Here's how the part is built. I have some questions about the finished solid (model axes, mm). A direction names the side the tool comes from. Coordinates: 2 decimals unless noted, no trailing zeros. Write each loop counter-clockwise with the first axis right and the second up, starting at its lowest first coordinate (ties: lowest second). Pieces come first, ordered by that corner, then holes. Notation, with made-up numbers: (76, -20.75) -> (120, -20.75) arc R9 ccw to (120, -9.75) -> close; hole circle Ø3 at (-26.75, -20). An arc over 180 degrees is marked (long way). Use CSV: the item, a comma, the result in double quotes. Start each with the question number.
```python
from build123d import *

# Parameters (mm, degrees)
SKETCH1_W               = 88.9
SKETCH1_H               = 40
BOSS_EXTRUDE1_DEPTH     = 20
SKETCH2_R               = 5
CUT_EXTRUDE1_DEPTH      = 89.9
SKETCH3_R               = 5.6
CUT_EXTRUDE2_DEPTH      = 10
SKETCH4_R               = 4
CUT_EXTRUDE3_DEPTH      = 10
F_1_4_20_TAPPED_HOLE1_D = 5.1054
CHAMFER1_SIZE           = 1


with BuildPart() as part:
    # Sketch1 → Boss-Extrude1 (new body)
    with BuildSketch(Plane(origin=(0, 0, 0), x_dir=(1, 0, 0), z_dir=(0, 1, 0))):
        Rectangle(SKETCH1_W, SKETCH1_H)
    extrude(amount=BOSS_EXTRUDE1_DEPTH)

    # Sketch2 → Cut-Extrude1 (cut, through all)
    with BuildSketch(Plane(origin=(44.45, 0, 0), x_dir=(0, 0, -1), z_dir=(1, 0, 0))):
        with Locations((-10, 10)):
            Circle(SKETCH2_R)
    extrude(amount=-CUT_EXTRUDE1_DEPTH, mode=Mode.SUBTRACT)

    # Sketch3 → Cut-Extrude2 (cut)
    with BuildSketch(Plane(origin=(44.45, 0, 0), x_dir=(0, 0, -1), z_dir=(1, 0, 0))):
        with Locations((-10, 10)):
            Circle(SKETCH3_R)
    cut_extrude2 = extrude(amount=-CUT_EXTRUDE2_DEPTH, mode=Mode.SUBTRACT)

    # Mirror1: Cut-Extrude2 across plane
    add(cut_extrude2.mirror(Plane(origin=(0, 0, 0), x_dir=(0, 0, 1), z_dir=(1, 0, 0))), mode=Mode.SUBTRACT)

    # Sketch4 → Cut-Extrude3 (cut)
    with BuildSketch(Plane(origin=(0, 0, -20), x_dir=(-1, 0, 0), z_dir=(0, 0, -1))):
        with Locations((-22.5, 10)):
            Circle(SKETCH4_R)
        with Locations((22.5, 10)):
            Circle(SKETCH4_R)
    extrude(amount=-CUT_EXTRUDE3_DEPTH, mode=Mode.SUBTRACT)

    # 1/4-20 Tapped Hole1 (through all)
    with Locations(Plane(origin=(0, 20, 0), x_dir=(1, 0, 0), z_dir=(0, 1, 0))):
        with Locations((39.45, 15), (-39.45, 15)):
            Hole(F_1_4_20_TAPPED_HOLE1_D / 2)

    # Chamfer1
    chamfer1_edges = [part.edges().sort_by_distance(p)[0] for p in [
        (-44.45, 20, 0),
        (0, 20, 20),
        (44.45, 20, 0),
        (0, 0, 20),
        (-44.45, 0, 0),
        (0, 0, -20),
        (44.45, 0, 0),
        (0, 20, -20),
        (44.45, 10, 20),
        (-44.45, 10, 20),
        (-44.45, 10, -20),
        (44.45, 10, -20),
    ]]
    chamfer(chamfer1_edges, length=CHAMFER1_SIZE)


solid = part.part
```
Item 1: I want a section at B-B on x = 39.45. Please give me the cut outline in (y, z), then the cut area to 3 significant figures.
Item 2: I want a section at C-C on y = 12.5. Count the separate pieces of the cut face and the enclosed holes in it, then the cut area to 3 significant figures.
Item 3: I want a section at D-D on x = -4.5. Please give me the cut outline in (y, z).
Item 4: I want a section at A-A on z = -15. Please give me the cut outline in (x, y), then the cut area to 3 significant figures.
Item 5: I'm going to push flat-ended pins straight in: pin 1 (6.5 mm diameter, centred on y = 10, z = 10, fed in from -X); pin 2 (5.5 mm diameter, centred on y = 11.5, z = 8, fed in from +X); pin 3 (2.5 mm diameter, centred on x = -23.5, y = 12, fed in from -Z). Where does each tip first touch, or does it pass through?
Item 6: If I drill on line 1 along Y through (x, z) = (5, 10); line 2 along Z through (x, y) = (19.5, 9.75); line 3 along Z through (x, y) = (-14.5, 9), over which ranges is the centre line in solid material (lowest first)?
Item 7: Thinking about a two-plate mould opening in Y: for faces 1 (the flat face through (34.45, 15, 12)), 2 (the flat face through (-1, 20, 0)), 3 (the cylindrical face through (-37.569, 9.86, -16.725)), which applies, +Y half, -Y half, draft (parallel to the pull), parting line (faces both ways), or undercut?
Item 8: Which directions (+Z, -Z, +X, -X, +Y, -Y) give clear straight access to the entire face, cutting with the end or side of a thin tool? Please do faces 4 (the cylindrical face through (-18.504, 10.176, -15.07)), 5 (the flat face through (-34.45, 15, 12)), 6 (the cylindrical face through (39.52, 5.03, 7.42)).
Geometry says:
1,outline,"(0, -19) -> (1, -20) -> (19, -20) -> (20, -19) -> (20, -17.55) -> (0, -17.55) -> close; (0, -12.45) -> (20, -12.45) -> (20, 19) -> (19, 20) -> (1, 20) -> (0, 19) -> close; hole circle Ø11.2 at (10, 10)"
1,area,"597 mm2"
2,separate pieces,"2"
2,enclosed holes,"2"
2,area,"2,590 mm2"
3,outline,"(0, -19) -> (1, -20) -> (19, -20) -> (20, -19) -> (20, 19) -> (19, 20) -> (1, 20) -> (0, 19) -> close; hole circle Ø10 at (10, 10)"
4,outline,"(-44.45, 1) -> (-43.45, 0) -> (-42, 0) -> (-42, 20) -> (-43.45, 20) -> (-44.45, 19) -> close; (-36.9, 0) -> (36.9, 0) -> (36.9, 20) -> (-36.9, 20) -> close; (42, 0) -> (43.45, 0) -> (44.45, 1) -> (44.45, 19) -> (43.45, 20) -> (42, 20) -> close; hole circle Ø8 at (-22.5, 10); hole circle Ø8 at (22.5, 10)"
4,area,"1,470 mm2"
5,pin 1,"through"
5,pin 2,"x = 34.45"
5,pin 3,"z = -10"
6,line 1,"0 to 5, 15 to 20"
6,line 2,"-10 to 5.01, 14.99 to 20"
6,line 3,"-20 to 5.1, 14.9 to 20"
7,face 1,"undercut"
7,face 2,"+Y half"
7,face 3,"draft"
8,face 4,"-Z"
8,face 5,"-X"
8,face 6,"+X"
